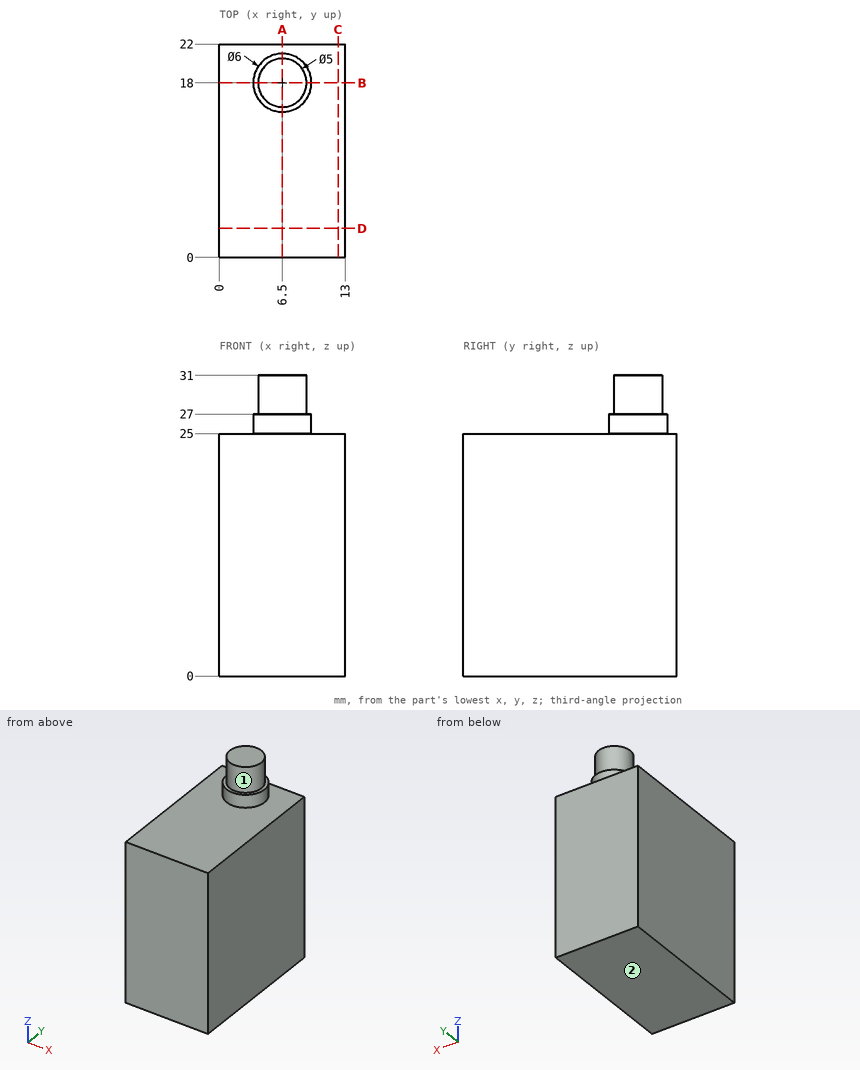
Geometry: see drawing. Coordinates: mm, zero at the bounding-box minimum. A direction names the side the tool comes from. Coordinates: 2 decimals unless noted, no trailing zeros. Loops run counter-clockwise (first coordinate to the right, second up) from the corner with the lowest first, then second, coordinate; pieces in that order, holes last.
Q1. Cut plane B-B (y = 18). Output: boundary loops of the cut face in (x, z), then the cut area to 3 significant figures.
Q2. Material intervals for line 1 (Z direction, x = 5, y = 12.75); line 2 (Y direction, x = 4, z = 26.5), sorted ascending.
Q3. Set-up query: the marked faces 1 and 2. Return all of +Z, -Z, +X, -X, +Y, -Y with unobstructed straight access to the full face (end or side cutting, diameter ignored); none if empty.
Q4. Cut plane D-D (y = 3). Output: boundary loops of the cut face in (x, z), then the cut area to 3 significant figures.
Q5. Cut plane A-A (x = 6.5). Output: boundary loops of the cut face in (y, z).
Q6. Cut plane C-C (x = 12.25). Output: boundary loops of the cut face in (y, z).
Working result:
1. outline: (0, 0) - (13, 0) - (13, 25) - (9.5, 25) - (9.5, 27) - (9, 27) - (9, 31) - (4, 31) - (4, 27) - (3.5, 27) - (3.5, 25) - (0, 25) - close
1. area: 357 mm2
2. line 1: z = 0 to 25
2. line 2: y = 16.34 to 19.66
3. face 1: +Z
3. face 2: -Z, +X, -X, +Y, -Y
4. outline: (0, 0) - (13, 0) - (13, 25) - (0, 25) - close
4. area: 325 mm2
5. outline: (0, 0) - (22, 0) - (22, 25) - (21, 25) - (21, 27) - (20.5, 27) - (20.5, 31) - (15.5, 31) - (15.5, 27) - (15, 27) - (15, 25) - (0, 25) - close
6. outline: (0, 0) - (22, 0) - (22, 25) - (0, 25) - close
